The listing builds one solid part. Answer for the finished solid, in the listing's coordinates (mm). Face numbers are marked on the shaded views. A direction names the side the tool comes from. Coordinates: 2 decimals unless noted, no trailing zeros. Write each loop counter-clockwise with the first axis right and the second up, starting at its lowest first coordinate (ties: lowest second). Pieces come first, ordered by that corner, then holes. Notation, with made-up numbers: M 56.5,-27.5 L 66.5,-27.5 A30 cw 66.5,-1.5 Z; hole C 79,64.5 d6. An arc over 180 degrees is marked long. Answer as CSV lines item,"result".
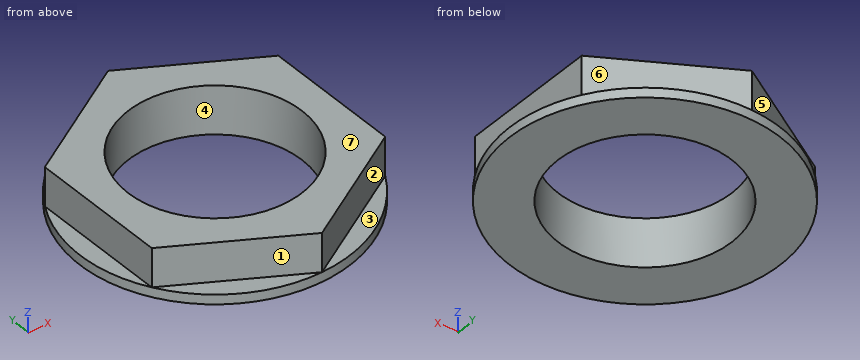
```python
from build123d import *

# Parameters (mm, degrees)
ESQUISSE1_R        = 7
ESQUISSE1_R_2      = 4.5
BOSS_EXTRU_1_DEPTH = 0.5
ESQUISSE2_R        = 4.5
BOSS_EXTRU_2_DEPTH = 2


with BuildPart() as part:
    # Esquisse1 → Boss.-Extru.1 (new body)
    with BuildSketch(Plane.XY):
        Circle(ESQUISSE1_R)
        Circle(ESQUISSE1_R_2, mode=Mode.SUBTRACT)
    extrude(amount=BOSS_EXTRU_1_DEPTH)

    # Esquisse2 → Boss.-Extru.2 (add)
    with BuildSketch(Plane.XY.offset(0.5)):
        Polygon((6.086240364, -3.457987599), (6.037825289, 3.541844969), (-0.048415075, 6.999832568), (-6.086240364, 3.457987599), (-6.037825289, -3.541844969), (0.048415075, -6.999832568), align=None)
        Circle(ESQUISSE2_R, mode=Mode.SUBTRACT)
    extrude(amount=BOSS_EXTRU_2_DEPTH)


solid = part.part
```
Q1. Find section D-D (x = -5.25). Give the vertices of the cut face in (y, z), and give its area (3 significant figures).
Output:
outline,"M -4.63,0 L 4.63,0 L 4.63,0.5 L 3.95,0.5 L 3.95,2.5 L -3.99,2.5 L -3.99,0.5 L -4.63,0.5 Z"
area,"20.5 mm2"
Q2. Straight lines are drawn through the part: line 1 (Z direction, x = 4.5, y = 5); line 2 (X direction, y = -2.25, z = 0.35); line 3 (Y direction, x = 1.25, z = 0.6). For each, find the intervals that lie inside material, in ascending order.
Output:
line 1,"0 to 0.5"
line 2,"-6.63 to -3.9, 3.9 to 6.63"
line 3,"-6.29 to -4.32, 4.32 to 6.26"
Q3. For the marked faces 5, 6 and 7, determine the directions among +Z, -Z, +X, -X, +Y, -Y from which every point of the face is accessible in a straight line to the end or side of a thin tool.
Output:
face 5,"+Z, -X, +Y"
face 6,"+Z, +X, +Y"
face 7,"+Z, +X, -X, +Y, -Y"
Q4. The mould has two halves that part along X. Classify the marked faces 1, 2, 3 and 4: pulls with the +X half, pulls with the -X half, needs draft (parallel to the pull), parting line crosses it, or undercut.
Output:
face 1,"pulls with the -X half"
face 2,"pulls with the +X half"
face 3,"needs draft"
face 4,"undercut"
Q5. Flat-ended cylindrical pins translate along their axes: pin 1 Ø1 at (y, z) = (3, 1.5) entering from +X; pin 2 Ø1.1 at (x, y) = (-3.5, 6) entering from +Z. Find the tip coordinate at first contact, or state that the pin passes through.
Output:
pin 1,"x = 6.05"
pin 2,"z = 0.5"
Q6. Find section A-A (z = 2.1). Give the vertices of the cut face in (x, y).
Output:
outline,"M -6.09,3.46 L -6.04,-3.54 L 0.05,-7 L 6.09,-3.46 L 6.04,3.54 L -0.05,7 Z; hole C 0,0 d9"
Q7. Find section B-B (x = 4.25). Give the vertices of the cut face in (y, z), and give its area (3 significant figures).
Output:
outline,"M -5.56,0 L -1.48,0 L -1.48,2.5 L -4.54,2.5 L -4.54,0.5 L -5.56,0.5 Z; M 1.48,0 L 5.56,0 L 5.56,0.5 L 4.56,0.5 L 4.56,2.5 L 1.48,2.5 Z"
area,"16.4 mm2"
Q8. Find section C-C (y = 1). Give the vertices of the cut face in (x, z).
Output:
outline,"M -6.93,0 L -4.39,0 L -4.39,2.5 L -6.07,2.5 L -6.07,0.5 L -6.93,0.5 Z; M 4.39,0 L 6.93,0 L 6.93,0.5 L 6.06,0.5 L 6.06,2.5 L 4.39,2.5 Z"
